Build history of the part. All positions in model axes, mm. Face numbers are marked on the shaded views. A direction names the side the tool comes from. Round coordinates to 2 decimals unless told otherwise and drop trailing zeros. Order: outer loops, then holes, each group sorted by start corner. A loop starts at its lowest first (then second) coordinate and runs counter-clockwise, first axis right, second up. Notation, with made-up numbers: M 71,-26.75 L 124,-26.75 A18 cw 124,-11.75 Z; hole C 4.5,43 d1. An arc over 180 degrees is marked long. One line per question, with ' | ' between items. Start each with the question number.
from build123d import *

# Parameters (mm, degrees)
F0_W     = 100
F0_H     = 80
F1_DEPTH = 8
F2_R     = 2.5
F3_DEPTH = 25
F4_W     = 100
F4_H     = 10
F5_DEPTH = 15
F6_R     = 2.526813
F7_DEPTH = 25
F8_R     = 7.5
F9_DEPTH = 25


with BuildPart() as f1:
    # F0 (on Top) → F1 (new body)
    with BuildSketch(Plane.XY):
        Rectangle(F0_W, F0_H)
    extrude(amount=F1_DEPTH)

    # F2 (on face) → F3 (cut)
    with BuildSketch(Plane.XY.offset(8)):
        with Locations((-32.754592, -11.921697)):
            Circle(F2_R)
        with Locations((-26.726142, -22.425896)):
            Circle(F2_R)
        with Locations((-17.5, -30.310889)):
            Circle(F2_R)
        with Locations((0, -35)):
            Circle(F2_R)
        with Locations((-35, 0)):
            Circle(F2_R)
        with Locations((17.5, -30.310889)):
            Circle(F2_R)
        with Locations((26.811556, -22.497566)):
            Circle(F2_R)
        with Locations((32.889242, -11.970705)):
            Circle(F2_R)
        with Locations((35, 0)):
            Circle(F2_R)
        with Locations((-9.058667, -33.807404)):
            Circle(F2_R)
        with Locations((9.058667, -33.807404)):
            Circle(F2_R)
    extrude(amount=-F3_DEPTH, mode=Mode.SUBTRACT)

    # F4 (on face) → F5 (join)
    with BuildSketch(Plane(origin=(0, 0, 0), x_dir=(1, 0, 0), z_dir=(0, 0, -1))):
        with Locations((0, -35)):
            Rectangle(F4_W, F4_H)
    extrude(amount=F5_DEPTH)

    # F6 (on face) → F7 (cut)
    with BuildSketch(Plane(origin=(0, 40, 0), x_dir=(-1, 0, 0), z_dir=(0, 1, 0))):
        with Locations((35, -5)):
            Circle(F6_R)
        with Locations((-35, -5)):
            Circle(F6_R)
    extrude(amount=-F7_DEPTH, mode=Mode.SUBTRACT)

    # F8 (on face) → F9 (cut)
    with BuildSketch(Plane.XY.offset(8)):
        with Locations((0, 20)):
            Circle(F8_R)
    extrude(amount=-F9_DEPTH, mode=Mode.SUBTRACT)


solid = f1.part
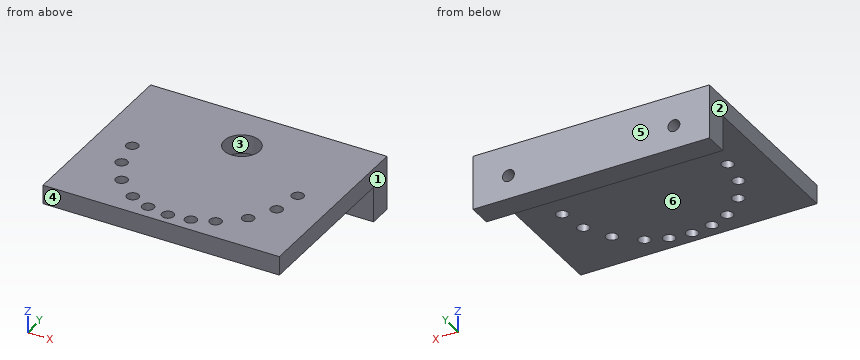
Item 1: Cut at C-C on y = 0. Write the cut outline in (x, z).
Item 2: Two-plate mould, pull along X, no slides. Class the marked faces 1, 2, 3 and 4: +X half, -X half, draft (parallel to the pull), parting line (faces both ways), or undercut.
Item 3: Flat gauge pins, fed straight in: pin 1 (8 mm diameter, centred on x = -17.5, y = -30.31, fed in from -Z); pin 2 (7.5 mm diameter, centred on x = -8.5, z = -10, fed in from -Y). Where does each tip first touch, or does it go through?
Item 4: Wall check: line 1 along Y through (x, z) = (0, 4); line 2 along Y through (x, z) = (-17.5, 2.25); line 3 along Z through (x, y) = (38, -30). Give the ranges that are in metal, low to high. Write a range as [from, to].
Item 5: Cut at A-A on x = -17.5. Write the cut outline in (y, z), then the cut area to 3 significant figures.
Item 6: Cut at B-B on y = 20. Write the cut outline in (x, z).
Item 7: Cut at D-D on z = -5. Write the cut outline in (x, y).
Item 8: Tool access for the marked faces 5 and 6: list every direction of +Z, -Z, +X, -X, +Y, -Y with a clear straight run to the whole face (end or side of a thin tool).
Results found:
1) outline: M -50,0 L -37.5,0 L -37.5,8 L -50,8 Z; M -32.5,0 L 32.5,0 L 32.5,8 L -32.5,8 Z; M 37.5,0 L 50,0 L 50,8 L 37.5,8 Z
2) face 1: +X half | face 2: -X half | face 3: undercut | face 4: draft
3) pin 1: stops at z = 0 | pin 2: stops at y = 30
4) line 1: y = [-40, -37.5], [-32.5, 12.5], [27.5, 40] | line 2: y = [-40, -32.81], [-27.81, 40] | line 3: z = [0, 8]
5) outline: M -40,0 L -32.81,0 L -32.81,8 L -40,8 Z; M -27.81,0 L 30,0 L 30,-15 L 40,-15 L 40,8 L -27.81,8 Z | area: 750 mm^2
6) outline: M -50,0 L -7.5,0 L -7.5,8 L -50,8 Z; M 7.5,0 L 50,0 L 50,8 L 7.5,8 Z
7) outline: M -50,30 L -37.53,30 L -37.53,40 L -50,40 Z; M -32.47,30 L 32.47,30 L 32.47,40 L -32.47,40 Z; M 37.53,30 L 50,30 L 50,40 L 37.53,40 Z
8) face 5: +Z, -Z, +X, -X, +Y | face 6: -Z, +X, -X, -Y
